Geometry check sheet. Reference: the model listing, model coordinates, mm. Face numbers are marked on the shaded views. A direction names the side the tool comes from. Coordinates: 2 decimals unless noted, no trailing zeros. Order: outer loops, then holes, each group sorted by start corner. A loop starts at its lowest first (then second) coordinate and runs counter-clockwise, first axis right, second up. Notation, with made-up numbers: (65.25, 85) - (86.25, 85) arc R21 ccw to (86.25, 122) - close; hole circle Ø11 at (19, 75). An arc over 180 degrees is marked (long way). Put each result on its own line as item: value.
from build123d import *

# Parameters (mm, degrees)
SKETCH_1_R               = 1.107438874
EXTRUDE_1_DEPTH          = 40
CUT_EXTRUDE_1_DEPTH      = 40
CUT_EXTRUDE_1_DEPTH_BACK = 40
SKETCH_3_W               = 4
SKETCH_3_H               = 8
CUT_EXTRUDE_2_DEPTH      = 10


with BuildPart() as part:
    # Sketch 1 → Extrude 1 (new body)
    with BuildSketch(Plane(origin=(0, 0, 0), x_dir=(1, 0, 0), z_dir=(0, 1, 0))):
        with BuildLine():
            ThreePointArc((-8, 1), (-11.414213562, 2.414213562), (-10, -1))
            Line((-10, -1), (10, -1))
            Line((10, -1), (10, 1))
            Line((10, 1), (-8, 1))
        make_face()
        with Locations(Location((-10, 1, 0), (0, 0, 270))):
            Circle(SKETCH_1_R, mode=Mode.SUBTRACT)
    extrude(amount=EXTRUDE_1_DEPTH)

    # Sketch 3 → Cut-Extrude 1 (cut, two sides: drawn at the far end of the back side and taken through both)
    with BuildSketch(Plane(origin=(0, 0, -1), x_dir=(-1, 0, 0), z_dir=(0, 0, -1)).offset(-CUT_EXTRUDE_1_DEPTH_BACK)):
        with Locations((10, 24)):
            Rectangle(SKETCH_3_W, SKETCH_3_H)
        with Locations((10, 16)):
            Rectangle(SKETCH_3_W, SKETCH_3_H)
    extrude(amount=CUT_EXTRUDE_1_DEPTH + CUT_EXTRUDE_1_DEPTH_BACK, mode=Mode.SUBTRACT)

    # Sketch 5 → Cut-Extrude 2 (cut)
    with BuildSketch(Plane(origin=(0, 0, -1), x_dir=(-1, 0, 0), z_dir=(0, 0, -1))):
        with BuildLine():
            ThreePointArc((0.5, 32.5), (-0.378679656, 34.621320344), (-2.5, 35.5))
            Line((-2.5, 35.5), (-2.5, 32.5))
            Line((-2.5, 32.5), (-5.5, 32.5))
            ThreePointArc((-5.5, 32.5), (-2.5, 29.5), (0.5, 32.5))
        make_face()
        with BuildLine():
            Line((-2.5, 32.5), (-2.5, 35.5))
            ThreePointArc((-2.5, 35.5), (-4.621320344, 34.621320344), (-5.5, 32.5))
            Line((-5.5, 32.5), (-2.5, 32.5))
        make_face()
        with BuildLine():
            ThreePointArc((-5.5, 7.5), (-4.621320344, 5.378679656), (-2.5, 4.5))
            Line((-2.5, 4.5), (-2.5, 7.5))
            Line((-2.5, 7.5), (-5.5, 7.5))
        make_face()
        with BuildLine():
            Line((-2.5, 7.5), (-2.5, 4.5))
            ThreePointArc((-2.5, 4.5), (-0.378679656, 5.378679656), (0.5, 7.5))
            ThreePointArc((0.5, 7.5), (-2.5, 10.5), (-5.5, 7.5))
            Line((-5.5, 7.5), (-2.5, 7.5))
        make_face()
    extrude(amount=-CUT_EXTRUDE_2_DEPTH, mode=Mode.SUBTRACT)


solid = part.part
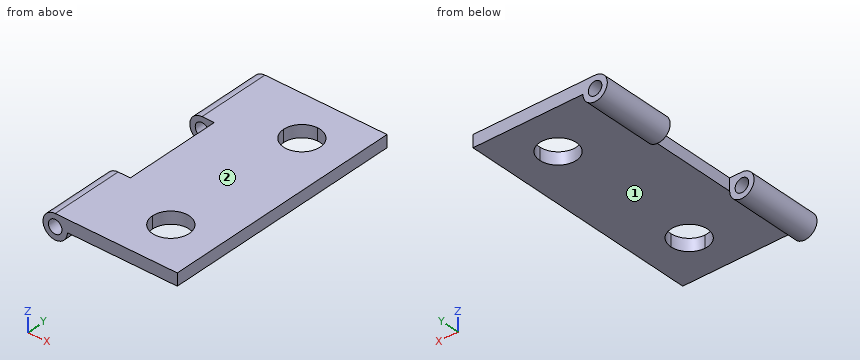
Q1. Thickness scan on L1, parallel to Z at x = -10, y = 6.5; L2, parallel to Y at x = 0.25, z = -0.95; L3, parallel to Y at x = -9.75, z = 0.85. Record the ranges inside material, lowest first. Write a range as [from, to].
Answer block:
L1: z = [-3, -2.11], [0.11, 1]
L2: y = [0, 5.52], [9.48, 30.52], [34.48, 40]
L3: y = [0, 12], [28, 40]
Q2. Access from +Z, -Z, +X, -X, +Y, -Y to the whole of each face (thin tool, end or side, straight path). Record for the marked faces 1 and 2.
Answer block:
face 1: -Z, +X, +Y, -Y
face 2: +Z, +X, -X, +Y, -Y
Q3. Section check D-D on x = 3.5. Record the boundary of the cut face in (y, z), then the cut area to 3 significant figures.
Answer block:
outline: (0, -1) - (4.67, -1) - (4.67, 1) - (0, 1) - close; (10.33, -1) - (29.67, -1) - (29.67, 1) - (10.33, 1) - close; (35.33, -1) - (40, -1) - (40, 1) - (35.33, 1) - close
area: 57.4 mm^2
Q4. Section check B-B on z = -0.6. Record the boundary of the cut face in (x, y), then the cut area to 3 significant figures.
Answer block:
outline: (-11.96, 0) - (-11.03, 0) - (-11.03, 12) - (-11.96, 12) - close; (-11.96, 28) - (-11.03, 28) - (-11.03, 40) - (-11.96, 40) - close; (-8.97, 0) - (10, 0) - (10, 40) - (-8.97, 40) - (-8.97, 28) - (-8, 28) - (-8, 12) - (-8.97, 12) - close; hole circle Ø6 at (2.5, 7.5); hole circle Ø6 at (2.5, 32.5)
area: 709 mm^2
Q5. Depth check by flat-ended pin: pin 1 Ø1.5 at (y, z) = (17, -2.5) entering from +X; pin 2 Ø0.6 at (y, z) = (23.5, 0) entering from -X; pin 3 Ø9 at (x, y) = (1.5, 27.5) entering from -Z. Enter the tip coordinate at first touch or a pass-through.
Answer block:
pin 1: passes through
pin 2: stops at x = -8
pin 3: stops at z = -1
Q6. Section check A-A on z = -2.6. Record the boundary of the cut face in (x, y).
Answer block:
outline: (-11.2, 0) - (-8.8, 0) - (-8.8, 12) - (-11.2, 12) - close; (-11.2, 28) - (-8.8, 28) - (-8.8, 40) - (-11.2, 40) - close
Q7. Section check C-C on y = 29. Record the boundary of the cut face in (x, z), then the cut area to 3 significant figures.
Answer block:
outline: (-10, 1) arc R2 ccw (long way) to (-8, -1) - (10, -1) - (10, 1) - close; hole circle Ø2.21 at (-10, -1)
area: 45.6 mm^2
